Part model, mm, in its own coordinate system. Coordinates: 2 decimals unless noted, no trailing zeros. Loops run counter-clockwise (first coordinate to the right, second up) from the corner with the lowest first, then second, coordinate; pieces in that order, holes last. Notation, with made-up numbers: (-34, 36.25) - (12, 36.25) arc R23 ccw to (12, 59.25) - close; hole circle Ø10 at (44.25, -4). An arc over 180 degrees is marked (long way). Answer as CSV lines item,"result".
from build123d import *

# Parameters (mm, degrees)
SKETCH2_R           = 4
SKETCH2_R_2         = 1.5
SKETCH2_R_3         = 0.75
BOSS_EXTRUDE1_DEPTH = 5


with BuildPart() as part:
    # Sketch2 → Boss-Extrude1 (new body)
    with BuildSketch(Plane.XY):
        with BuildLine():
            Line((12.5, 0), (12.5, -110))
            ThreePointArc((12.5, -110), (0, -122.5), (-12.5, -110))
            Line((-12.5, -110), (-12.5, 0))
            ThreePointArc((-12.5, 0), (0, 12.5), (12.5, 0))
        make_face()
        Circle(SKETCH2_R, mode=Mode.SUBTRACT)
        with Locations((0, -110)):
            Circle(SKETCH2_R, mode=Mode.SUBTRACT)
        with Locations((7, -47.5)):
            Circle(SKETCH2_R_2, mode=Mode.SUBTRACT)
        with Locations((-7, -47.5)):
            Circle(SKETCH2_R_2, mode=Mode.SUBTRACT)
        with Locations((7, -62.5)):
            Circle(SKETCH2_R_2, mode=Mode.SUBTRACT)
        with Locations((-7, -62.5)):
            Circle(SKETCH2_R_2, mode=Mode.SUBTRACT)
        with Locations((6.390950113, -110.266167545)):
            Circle(SKETCH2_R_3, mode=Mode.SUBTRACT)
        with Locations((-0.266167545, -116.390950113)):
            Circle(SKETCH2_R_3, mode=Mode.SUBTRACT)
        with Locations((-6.390950113, -109.733832455)):
            Circle(SKETCH2_R_3, mode=Mode.SUBTRACT)
        with Locations((0.266167545, -103.609049887)):
            Circle(SKETCH2_R_3, mode=Mode.SUBTRACT)
        with Locations((-6.396483965, 0.009022015)):
            Circle(SKETCH2_R_3, mode=Mode.SUBTRACT)
        with Locations((0.009022015, 6.396483965)):
            Circle(SKETCH2_R_3, mode=Mode.SUBTRACT)
        with Locations((-0.009022015, -6.396483966)):
            Circle(SKETCH2_R_3, mode=Mode.SUBTRACT)
        with Locations((6.396483965, -0.009022016)):
            Circle(SKETCH2_R_3, mode=Mode.SUBTRACT)
    extrude(amount=BOSS_EXTRUDE1_DEPTH)


solid = part.part
Q1. Saw through at A-A (y = -47.5). Give the cut face in (x, z).
Results:
outline,"(-12.5, 0) - (-8.5, 0) - (-8.5, 5) - (-12.5, 5) - close; (-5.5, 0) - (5.5, 0) - (5.5, 5) - (-5.5, 5) - close; (8.5, 0) - (12.5, 0) - (12.5, 5) - (8.5, 5) - close"
Q2. Saw through at B-B (z = 3.6). Count the separate pieces of the cut face and the enclosed holes in it, then the cut area to 3 significant figures.
Results:
separate pieces,"1"
enclosed holes,"14"
area,"3,100 mm^2"
Q3. Two-plate mould, pull along Y, no slides. Class faces 1 (the face through (-0.275, 12.497, 2.465)), 2 (the face through (0, -54, 5)), 3 (the face through (-0.867, -3.905, 2.465)): released by +Y, released by -Y, zero draft, split by the parting line, or undercut.
Results:
face 1,"released by +Y"
face 2,"zero draft"
face 3,"undercut"
Q4. Wall check: L1, parallel to Y at x = 5.75, z = 0.7; L2, parallel to Y at x = 6.75, z = 4.5; L3, parallel to X at y = -48, z = 3.7. Give the ranges that are in metal, low to high.
Results:
L1,"y = -121.1 to -110.66, -109.88 to -63.33, -61.67 to -48.33, -46.67 to -0.39, 0.37 to 11.1"
L2,"y = -120.52 to -110.92, -109.61 to -63.98, -61.02 to -48.98, -46.02 to -0.67, 0.65 to 10.52"
L3,"x = -12.5 to -8.41, -5.59 to 5.59, 8.41 to 12.5"
